from build123d import *

# Parameters (mm, degrees)
F1_W     = 152.4
F1_H     = 152.4
F2_DEPTH = 76.2
F3_W     = 76.2
F3_H     = 76.2
F4_DEPTH = 76.201


# Not quite as in the source:
# - a variable given as a bare number and used for a length is read in inches; the dataset says mm whatever the document's units were


with BuildPart() as f2:
    # F1 (on Front) → F2 (new body)
    with BuildSketch(Plane.XZ):
        Rectangle(F1_W, F1_H)
    extrude(amount=F2_DEPTH)

    # F3 (on face) → F4 (cut, through all)
    with BuildSketch(Plane.XZ.offset(76.2)):
        with Locations((38.1, -38.1)):
            Rectangle(F3_W, F3_H)
    extrude(amount=-F4_DEPTH, mode=Mode.SUBTRACT)


solid = f2.part
The listing builds one solid part. Answer for the finished solid, in the listing's coordinates (mm). A direction names the side the tool comes from. Give positions to 0.01 mm unless a question says otherwise; leave off trailing zeros. Write each loop counter-clockwise with the first axis right and the second up, starting at its lowest first coordinate (ties: lowest second). Pieces come first, ordered by that corner, then holes. Notation, with made-up numbers: (17.5, 10.5) - (57.5, 10.5) arc R12 cw to (57.5, 32.5) - close; hole circle Ø5 at (40, -5.5). An arc over 180 degrees is marked (long way). Use a Markdown table: item, result.
1. Section B-B on x = 27 is taken. Write down the section's boundary in (y, z).
Values follow:
| item | result |
|---|---|
| outline | (-76.2, 0) - (0, 0) - (0, 76.2) - (-76.2, 76.2) - close |
2. Section A-A on y = -27 is taken. Write down the section's boundary in (x, z).
Values follow:
| item | result |
|---|---|
| outline | (-76.2, -76.2) - (0, -76.2) - (0, 0) - (76.2, 0) - (76.2, 76.2) - (-76.2, 76.2) - close |
3. A tool of negligible diameter and unlimited length cuts with its end or side. For faces 1 (the flat face through (38, -39, 0)), 2 (the flat face through (-18, 0, 18)), from which of +Z, -Z, +X, -X, +Y, -Y can it reach the whole face along a straight path? Write none if from no direction.
Values follow:
| item | result |
|---|---|
| face 1 | -Z, +X, +Y, -Y |
| face 2 | +Z, -Z, +X, -X, +Y |
4. Find the intervals of material crossed by probe 1 along Z at (x, y) = (67, -66.5); probe 2 along X at (y, z) = (-34, -28), in increasing order. Write a range as from..to.
Values follow:
| item | result |
|---|---|
| probe 1 | z = 0..76.2 |
| probe 2 | x = -76.2..0 |
5. Section C-C on z = -41 is taken. Write down the section's boundary in (x, y).
Values follow:
| item | result |
|---|---|
| outline | (-76.2, -76.2) - (0, -76.2) - (0, 0) - (-76.2, 0) - close |
